from build123d import *

# Parameters (mm, degrees)
BOSS_EXTRUDE1_DEPTH = 1.5875
BOSS_EXTRUDE2_DEPTH = 1.5875
SKETCH5_R           = 3.81
CUT_EXTRUDE1_DEPTH  = 3.175


with BuildPart() as part:
    # Sketch3 → Boss-Extrude1 (new, symmetric)
    with BuildSketch(Plane.YZ):
        Polygon((-19.8628, 0), (-19.8628, 3.175), (-15.86484, 3.175), (-15.86484, 12.7), (15.86484, 12.7), (15.86484, 3.175), (21.4122, 3.175), (21.4122, 0), (12.5984, 0), (12.5984, 7.0612), (-12.5984, 7.0612), (-12.5984, 0), align=None)
    extrude(amount=BOSS_EXTRUDE1_DEPTH, both=True)

    # Sketch4 → Boss-Extrude2 (add, symmetric)
    with BuildSketch(Plane.YZ):
        with BuildLine():
            Line((-14.224, 12.7), (-14.224, 15.875))
            ThreePointArc((-14.224, 15.875), (0, 30.099), (14.224, 15.875))
            Line((14.224, 15.875), (14.224, 12.7))
            Line((14.224, 12.7), (15.86484, 12.7))
            Line((15.86484, 12.7), (15.86484, 3.175))
            Line((15.86484, 3.175), (21.4122, 3.175))
            Line((21.4122, 3.175), (21.4122, 0))
            Line((21.4122, 0), (12.5984, 0))
            Line((12.5984, 0), (12.5984, 7.0612))
            Line((12.5984, 7.0612), (-12.5984, 7.0612))
            Line((-12.5984, 7.0612), (-12.5984, 0))
            Line((-12.5984, 0), (-19.8628, 0))
            Line((-19.8628, 0), (-19.8628, 3.175))
            Line((-19.8628, 3.175), (-15.86484, 3.175))
            Line((-15.86484, 3.175), (-15.86484, 12.7))
            Line((-15.86484, 12.7), (-14.224, 12.7))
        make_face()
    extrude(amount=BOSS_EXTRUDE2_DEPTH, both=True)

    # Sketch5 → Cut-Extrude1 (cut)
    with BuildSketch(Plane.YZ.offset(1.5875)):
        with Locations(Location((0, 22.873624204, 0), (0, 0, 270))):
            Circle(SKETCH5_R)
    extrude(amount=-CUT_EXTRUDE1_DEPTH, mode=Mode.SUBTRACT)


solid = part.part
Build history of the part. All positions in model axes, mm. A direction names the side the tool comes from. Round coordinates to 2 decimals unless told otherwise and drop trailing zeros. Write each loop counter-clockwise with the first axis right and the second up, starting at its lowest first coordinate (ties: lowest second). Pieces come first, ordered by that corner, then holes. Notation, with made-up numbers: M 82,69.5 L 98,69.5 A22 ccw 98,108.5 Z; hole C 56.5,21.5 d1. An arc over 180 degrees is marked long. Answer in a Markdown table with one row per item.
1. Probe L1, parallel to Y at x = 0.05, z = 1.5; L2, parallel to Y at x = 1.4, z = 14.5; L3, parallel to Z at x = 0, y = -16 (3 decimals). List the from-to ranges inside material, lowest first. Write a range as [from, to].
Geometry check:
| item | result |
|---|---|
| L1 | [-19.86, -12.6], [12.6, 21.41] |
| L2 | [-14.22, 14.22] |
| L3 | [0, 3.175] |
2. Flat gauge pins, fed straight in: P1, Ø1.3, axis at x = -0.5, y = -15, coming from the +Z side; P2, Ø1, axis at x = 1, y = -18.5, coming from the +Z side (3 decimals); P3, Ø1.6, axis at x = 0.5, z = 9.5, coming from the -Y side. Where does each tip first touch, or does it go through?
Geometry check:
| item | result |
|---|---|
| P1 | z = 12.7 |
| P2 | z = 3.175 |
| P3 | y = -15.86 |
3. Mould opens along Z. For faces 5 (the face through (0, -19.863, 2)), 6 (the face through (0, -15, 12.7)), 7 (the face through (0.02, 1.14, 19.24)) say: +Z half, -Z half, draft (parallel to the pull), parting line (faces both ways), or undercut.
Geometry check:
| item | result |
|---|---|
| face 5 | draft |
| face 6 | +Z half |
| face 7 | undercut |
4. Saw through at B-B (x = 0.2). List the corners of the cut face in (y, z) (3 decimals).
Geometry check:
| item | result |
|---|---|
| outline | M -19.863,0 L -12.598,0 L -12.598,7.061 L 12.598,7.061 L 12.598,0 L 21.412,0 L 21.412,3.175 L 15.865,3.175 L 15.865,12.7 L 14.224,12.7 L 14.224,15.875 A14.224 ccw -14.224,15.875 L -14.224,12.7 L -15.865,12.7 L -15.865,3.175 L -19.863,3.175 Z; hole C 0,22.874 d7.62 |
5. Saw through at A-A (y = 0). List the corners of the cut face in (x, z), and give its area (3 significant figures).
Geometry check:
| item | result |
|---|---|
| outline | M -1.59,7.06 L 1.59,7.06 L 1.59,19.06 L -1.59,19.06 Z; M -1.59,26.68 L 1.59,26.68 L 1.59,30.1 L -1.59,30.1 Z |
| area | 49.0 mm2 |
6. Which spindle directions (+Z, -Z, +X, -X, +Y, -Y) get a long thin tool onto all of the face, cutting with end or side? Do faces 1 (the face through (0, 15, 12.7)), 2 (the face through (-1.588, 1, 15)), 3 (the face through (0, 0, 7.061)), 4 (the face through (0, -18, 3.175)). Say none if no direction does.
Geometry check:
| item | result |
|---|---|
| face 1 | +Z, +X, -X, +Y |
| face 2 | +Z, -Z, -X, +Y, -Y |
| face 3 | -Z, +X, -X |
| face 4 | +Z, +X, -X, -Y |
7. Saw through at D-D (y = -7). List the corners of the cut face in (x, z).
Geometry check:
| item | result |
|---|---|
| outline | M -1.59,7.06 L 1.59,7.06 L 1.59,28.26 L -1.59,28.26 Z |
8. Saw through at C-C (z = 7.5). List the corners of the cut face in (x, y), and give its area (3 significant figures).
Geometry check:
| item | result |
|---|---|
| outline | M -1.59,-15.86 L 1.59,-15.86 L 1.59,15.86 L -1.59,15.86 Z |
| area | 101 mm2 |
